```python
from build123d import *

# Parameters (mm, degrees)
BASE_EXTRUDE_DEPTH = 9.525
SKETCH4_R          = 4.7625
CUT_EXTRUDE1_DEPTH = 751.113488497


with BuildPart() as part:
    # Sketch1 → Base-Extrude (new body)
    with BuildSketch(Plane.XY.offset(130.175)):
        with BuildLine():
            Line((-114.134574641, 649.743144285), (-153.061701436, 410.92742286))
            ThreePointArc((-153.061701436, 410.92742286), (-156.988617271, 398.001466727), (-164.183568949, 386.567583735))
            Line((-164.183568949, 386.567583735), (-352.654107763, 160.533104066))
            ThreePointArc((-352.654107763, 160.533104066), (-354.840836834, 156.72509141), (-355.6, 152.4))
            Line((-355.6, 152.4), (-355.6, 139.7))
            Line((-355.6, 139.7), (-95.25, 139.7))
            ThreePointArc((-95.25, 139.7), (0, 234.95), (95.25, 139.7))
            Line((95.25, 139.7), (355.6, 139.7))
            Line((355.6, 139.7), (355.6, 152.4))
            ThreePointArc((355.6, 152.4), (354.840836834, 156.72509141), (352.654107763, 160.533104066))
            Line((352.654107763, 160.533104066), (164.183568949, 386.567583735))
            ThreePointArc((164.183568949, 386.567583735), (156.988617271, 398.001466727), (153.061701436, 410.92742286))
            Line((153.061701436, 410.92742286), (114.134574641, 649.743144285))
            ThreePointArc((114.134574641, 649.743144285), (109.826240562, 657.375689444), (101.6, 660.4))
            Line((101.6, 660.4), (-101.6, 660.4))
            ThreePointArc((-101.6, 660.4), (-109.826240562, 657.375689444), (-114.134574641, 649.743144285))
        make_face()
    extrude(amount=BASE_EXTRUDE_DEPTH)

    # Sketch4 → Cut-Extrude1 (cut, through all)
    with BuildSketch(Plane.XY.offset(139.7)):
        with Locations((0, 374.65)):
            Circle(SKETCH4_R)
        with Locations((114.3, 150.8252)):
            Circle(SKETCH4_R)
        with Locations(Location((-114.3, 150.8252, 0), (0, 0, 180))):
            Circle(SKETCH4_R)
    extrude(amount=-CUT_EXTRUDE1_DEPTH, mode=Mode.SUBTRACT)


solid = part.part
```
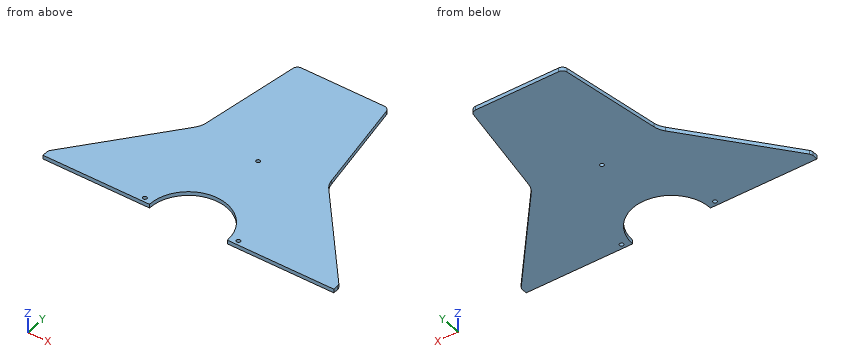
Model file for the job. Use its own axes, mm. Give positions to 0.01 mm unless a question says otherwise; leave off trailing zeros. Loops run counter-clockwise (first coordinate to the right, second up) from the corner with the lowest first, then second, coordinate; pieces in that order, holes last. Notation, with made-up numbers: (8.5, -37) -> (63.5, -37) arc R23 cw to (63.5, -2) -> close; hole circle Ø11 at (86.5, -10). An arc over 180 degrees is marked (long way). Write each question's results on one line, items separated by ' | '.
(1) Cut at B-B on x = -288.5. List the corners of the cut face in (y, z) (3 decimals).
Geometry results:
outline: (139.7, 130.175) -> (237.474, 130.175) -> (237.474, 139.7) -> (139.7, 139.7) -> close
(2) Probe line 1 along X through (y, z) = (371, 137); line 2 along Y through (x, z) = (-110, 134.5); line 3 along Y through (x, z) = (15.5, 134). List the from-to ranges inside material, lowest first.
Geometry results:
line 1: x = -177.16 to -3.06, 3.06 to 177.16 | line 2: y = 139.7 to 148.78, 152.87 to 657.23 | line 3: y = 233.68 to 660.4
(3) Cut at A-A on z = 133. Give the number of separate pieces and of enclosed holes in the cut face, and give its area (3 significant figures).
Geometry results:
separate pieces: 1 | enclosed holes: 3 | area: 191,000 mm²
(4) Flat gauge pins, fed straight in: pin 1 Ø4 at (y, z) = (248.5, 136.5) entering from -X; pin 2 Ø5 at (y, z) = (503, 134) entering from -X. Where does each tip first touch, or does it go through?
Geometry results:
pin 1: stops at x = -280.97 | pin 2: stops at x = -138.46
(5) Cut at C-C on y = 443. List the corners of the cut face in (x, z) (3 decimals), and give its area (3 significant figures).
Geometry results:
outline: (-147.834, 130.175) -> (147.834, 130.175) -> (147.834, 139.7) -> (-147.834, 139.7) -> close | area: 2,820 mm²
